```python
from build123d import *

# Parameters (mm, degrees)
SKETCH2_W           = 40
SKETCH2_H           = 40
SKETCH2_R           = 7
SKETCH2_R_2         = 1.5
BOSS_EXTRUDE1_DEPTH = 2
FILLET1_R           = 4


with BuildPart() as part:
    # Sketch2 → Boss-Extrude1 (new body)
    with BuildSketch(Plane(origin=(0, 0, 0), x_dir=(1, 0, 0), z_dir=(0, 1, 0))):
        Rectangle(SKETCH2_W, SKETCH2_H)
        Circle(SKETCH2_R, mode=Mode.SUBTRACT)
        with Locations((-9, 12)):
            Circle(SKETCH2_R_2, mode=Mode.SUBTRACT)
        with Locations((-9, -14.3)):
            Circle(SKETCH2_R_2, mode=Mode.SUBTRACT)
        with Locations((10.8, -14.3)):
            Circle(SKETCH2_R_2, mode=Mode.SUBTRACT)
        with Locations((10.8, 12)):
            Circle(SKETCH2_R_2, mode=Mode.SUBTRACT)
    extrude(amount=BOSS_EXTRUDE1_DEPTH)

    # Fillet1
    fillet1_edges = [part.edges().sort_by_distance(p)[0] for p in [
        (20, 1, 20),
        (-20, 1, 20),
        (-20, 1, -20),
        (20, 1, -20),
    ]]
    fillet(fillet1_edges, radius=FILLET1_R)


solid = part.part
```
CAD build for the part. Positions are in the model's coordinates, mm. Round coordinates to 2 decimals unless told otherwise and drop trailing zeros. Write each loop counter-clockwise with the first axis right and the second up, starting at its lowest first coordinate (ties: lowest second). Pieces come first, ordered by that corner, then holes. Notation, with made-up numbers: (25.5, 13.25) -> (39.5, 13.25) arc R21 cw to (39.5, 48.25) -> close; hole circle Ø8 at (6.5, 67). An arc over 180 degrees is marked (long way). Answer in a Markdown table with one row per item. Add a question column.
Item 1: Saw through at D-D, the plane x = 1. Write the cut outline in (y, z).
Item 2: Drop a flat-ended pin along its axis: pin 1 Ø1 at (x, z) = (15.5, -0.5) entering from -Y. Give the stop position or say it passes through.
Item 3: Saw through at C-C, the plane y = 1.1. Write the cut outline in (x, z).
Item 4: Saw through at B-B, the plane z = -6. Write the cut outline in (x, y), then the cut area to 3 significant figures.
Item 5: Drill centre lines: line 1 (Z direction, x = 10.8, y = 1.15); line 2 (X direction, y = 1.25, z = 14.3); line 3 (Z direction, x = 0, y = 0.35). Where is each one in solid material? Low to high. Write a range as from..to.
Item 6: Mould opens along Z. For faces 1 (the face through (0, 2, -9)), 2 (the face through (18.797, 1.014, 18.859)), 3 (the face through (-10.2, 1, 15.2)), 4 (the face through (12.186, 0.986, 14.875)) say: pulls with the +Z half, pulls with the -Z half, needs draft (parallel to the pull), parting line crosses it, or undercut.
Item 7: Saw through at A-A, the plane x = 10.8. Write the cut outline in (y, z), then the cut area to 3 significant figures.
Findings below:
| question | item | result |
|---|---|---|
| 1 | outline | (0, -20) -> (2, -20) -> (2, -6.93) -> (0, -6.93) -> close; (0, 6.93) -> (2, 6.93) -> (2, 20) -> (0, 20) -> close |
| 2 | pin 1 | stops at y = 0 |
| 3 | outline | (-20, -16) arc R4 ccw to (-16, -20) -> (16, -20) arc R4 ccw to (20, -16) -> (20, 16) arc R4 ccw to (16, 20) -> (-16, 20) arc R4 ccw to (-20, 16) -> close; hole circle Ø3 at (-9, -12); hole circle Ø3 at (-9, 14.3); hole circle Ø14 at (0, 0); hole circle Ø3 at (10.8, -12); hole circle Ø3 at (10.8, 14.3) |
| 4 | outline | (-20, 0) -> (-3.61, 0) -> (-3.61, 2) -> (-20, 2) -> close; (3.61, 0) -> (20, 0) -> (20, 2) -> (3.61, 2) -> close |
| 4 | area | 65.6 mm^2 |
| 5 | line 1 | z = -20..-13.5, -10.5..12.8, 15.8..20 |
| 5 | line 2 | x = -20..-10.5, -7.5..9.3, 12.3..20 |
| 5 | line 3 | z = -20..-7, 7..20 |
| 6 | face 1 | needs draft |
| 6 | face 2 | pulls with the +Z half |
| 6 | face 3 | undercut |
| 6 | face 4 | undercut |
| 7 | outline | (0, -20) -> (2, -20) -> (2, -13.5) -> (0, -13.5) -> close; (0, -10.5) -> (2, -10.5) -> (2, 12.8) -> (0, 12.8) -> close; (0, 15.8) -> (2, 15.8) -> (2, 20) -> (0, 20) -> close |
| 7 | area | 68.0 mm^2 |
